Here's how the part is built. I have some questions about the finished solid (model axes, mm). Face numbers are marked on the shaded views. Coordinates: 2 decimals unless noted, no trailing zeros. Order: outer loops, then holes, each group sorted by start corner. A loop starts at its lowest first (then second) coordinate and runs counter-clockwise, first axis right, second up. Notation, with made-up numbers: (17, -20) - (62, -20) arc R13 cw to (62, -15) - close; hole circle Ø1 at (74, 58). An arc over 180 degrees is marked (long way). Answer as CSV lines item,"result". Start each with the question number.
Item 1: Imagine slicing it at B-B on y = 15.75. List the corners of the cut face in (x, z) for me.
Item 2: I need wall thicknesses on line 1 (X direction, y = 10, z = 3); line 2 (X direction, y = 10, z = 1.65); line 3 (X direction, y = 1, z = 18). Which ranges of each line are inside material? Lowest first, please.
Item 3: Imagine slicing it at A-A on x = 0. List the corners of the cut face in (y, z) for me, and give its area (3 significant figures).
Item 4: I'm going to push flat-ended pins straight in: pin 1 (4 mm diameter, centred on x = -49, y = 13, fed in from +Z); pin 2 (6 mm diameter, centred on x = -26, y = 12.5, fed in from -Z) (3 decimals); pin 3 (4 mm diameter, centred on x = 50.5, y = 10, fed in from +Z). Where does each tip first touch, or does it pass through?
Item 5: We'd pull the mould along X, two halves only. Please class the marked faces 1, 2 and 3: pulls with the +X half, pulls with the -X half, needs draft (parallel to the pull), parting line crosses it, or undercut.
Autodesk Inventor part; units mm, degrees
ref_plane "Work Plane1" through (-42.5, 0, 0) normal (1, 0, 0) x (0, 1, 0)
ref_plane "XZ Plane" through (0, 0, 0) normal (0, 1, 0) x (-1, 0, 0)
ref_plane "XY Plane" through (0, 0, 0) normal (0, 0, 1) x (1, 0, 0)
sketch "Sketch1" plane through (0, 0, 0) normal (0, 1, 0) x (-1, 0, 0)
  circle A0 centre (0, 0) radius 42.5
  dimension "d0" = 85
extrude "Extrusion1" add sketch "Sketch1" along normal blind 20
shell "Shell1" thickness 5 removed faces 2 at (10.6049, 20, 7.3037) at (10.6049, 0, 7.3037)
sketch "Sketch2" plane through (0, 20, 0) normal (0, 1, 0) x (1, 0, 0)
  line L0 (-62.0625, 51.3519) -> (57.6609, 51.3519)
  line L1 (57.6609, 51.3519) -> (57.6609, 0)
  line L2 (57.6609, 0) -> (-62.0625, 0)
  line L3 (-62.0625, 0) -> (-62.0625, 51.3519)
  point P0 (0, 0)
extrude "Extrusion2" cut sketch "Sketch2" against normal through all
ref_plane "Work Plane1" through (-42.5, 0, 0) normal (1, 0, 0) x (0, 1, 0)
sketch "Sketch3" plane through (-42.5, 0, 0) normal (1, 0, 0) x (0, 1, 0)
  line L0 (0, 0) -> (0, 42.5)
  line L1 (0, 0) -> (20, 0)
  line L2 (20, 0) -> (20, 10)
  line L3 (20, 10) -> (0, 10)
  line L4 (0, 10) -> (0, 0)
  point P0 (0, 10)
  dimension "d7" = 20
  dimension "d8" = 10
extrude "Extrusion3" add sketch "Sketch3" along normal blind 2 and the other way blind 15
mirror "Mirror1" about plane through (0, 0, 0) normal (1, 0, 0) of "Extrusion3"
sketch "Sketch6" plane through (-57.5, 20, 10) normal (0, 0, 1) x (1, 0, 0)
  line L0 (10.3965, -14.0055) -> (5.7777, -13.9945)
  line L1 (5.7777, -13.9945) -> (3.4778, -9.9891)
  line L2 (3.4778, -9.9891) -> (5.7967, -5.9945)
  line L3 (5.7967, -5.9945) -> (10.4155, -6.0055)
  line L4 (10.4155, -6.0055) -> (12.7154, -10.0109)
  line L5 (12.7154, -10.0109) -> (10.3965, -14.0055)
  line L6 (0, -20) -> (0, 0)
  line L7 (0, 0) -> (16.1932, 0)
  point P0 (57.5, -20)
  point P1 (8.0966, -10)
  point P2 (0, -10)
  point P3 (8.0966, 0)
  dimension "d27" = 8
extrude "Extrusion4" cut sketch "Sketch6" against normal blind 5
sketch "Sketch7" plane through (-57.5, 20, 5) normal (0, 0, 1) x (1, 0, 0)
  line L0 (0, -20) -> (0, 0)
  line L1 (0, 0) -> (16.1932, 0)
  point P0 (57.5, -20)
  point P1 (8.0966, -10)
  point P2 (0, -10)
  point P3 (8.0966, 0)
hole "Hole3" at (-49.4034, 10, 5) direction (0, 0, -1) diameter 5.5 end through all
mirror "Mirror3" about plane through (0, 0, 0) normal (1, 0, 0) of "Extrusion4", "Hole3"
fillet "Fillet1" radius 2 23 edges at (-57.5, 0, 5) (-57.5, 20, 5) (-41.3068, 10, 10) (-49.4034, 0, 10) (-57.5, 10, 10) (-49.4034, 20, 10) (0, 20, 42.5) (0, 20, 37.5) (0, 0, 42.5) (-47.5, 20, 0) (47.5, 20, 0) (-57.5, 10, 0) (-47.5, 0, 0) (47.5, 0, 0) (0, 0, 37.5) (49.4034, 20, 10) (57.5, 10, 10) (49.4034, 0, 10) (57.5, 0, 5) (57.5, 20, 5) (57.5, 10, 0) (-37.5, 10, 0) (37.5, 10, 0)
properties part number "ur5e_cable_tube_bottom_75mm"
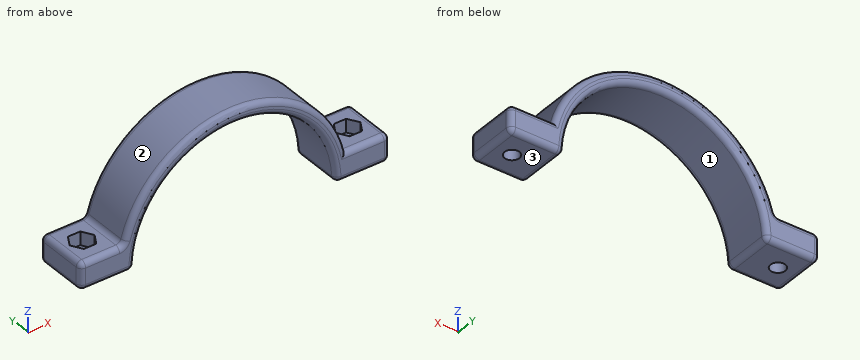
Responses:
1,outline,"(-57.5, 2) arc R2 ccw to (-55.5, 0) - (-39.45, 0) arc R2 ccw to (-37.45, 1.9) arc R37.5 cw to (37.45, 1.9) arc R2 ccw to (39.45, 0) - (55.5, 0) arc R2 ccw to (57.5, 2) - (57.5, 8) arc R2 ccw to (55.5, 10) - (41.31, 10) arc R42.5 ccw to (-40.93, 11.46) arc R2 cw to (-42.85, 10) - (-55.5, 10) arc R2 ccw to (-57.5, 8) - close"
2,line 1,"x = -57.5 to -52.15, -46.65 to -37.38, 37.38 to 46.65, 52.15 to 57.5"
2,line 2,"x = -57.47 to -52.15, -46.65 to -37.48, 37.48 to 46.65, 52.15 to 57.47"
2,line 3,"x = -38.2 to -33.2, 33.2 to 38.2"
3,outline,"(0, 39.5) arc R2 ccw to (2, 37.5) - (18, 37.5) arc R2 ccw to (20, 39.5) - (20, 40.5) arc R2 ccw to (18, 42.5) - (2, 42.5) arc R2 ccw to (0, 40.5) - close"
3,area,"96.6 mm^2"
4,pin 1,"stops at z = 10"
4,pin 2,"stops at z = 23.775"
4,pin 3,"stops at z = 5"
5,face 1,"undercut"
5,face 2,"parting line crosses it"
5,face 3,"needs draft"
